```python
from build123d import *

# Parameters (mm, degrees)
SKETCH_1_R          = 28.4
EXTRUDE_1_DEPTH     = 2
SKETCH_2_R          = 13.75
EXTRUDE_2_DEPTH     = 14
SKETCH_3_R          = 3.5
SKETCH_3_R_2        = 1.6
CUT_EXTRUDE_1_DEPTH = 44.233320483
SKETCH_4_R          = 2.1
CUT_EXTRUDE_2_DEPTH = 43.533751304


with BuildPart() as part:
    # ｽｹｯﾁ1 → ﾎﾞｽ - 押し出し1 (new body)
    with BuildSketch(Plane(origin=(0, 0, 0), x_dir=(1, 0, 0), z_dir=(0, 1, 0))):
        with Locations(Location((0, 0, 0), (0, 0, 270))):
            Circle(SKETCH_1_R)
    extrude(amount=EXTRUDE_1_DEPTH)

    # ｽｹｯﾁ2 → ﾎﾞｽ - 押し出し2 (add)
    with BuildSketch(Plane(origin=(0, 2, 0), x_dir=(1, 0, 0), z_dir=(0, 1, 0))):
        with Locations(Location((0, 0, 0), (0, 0, 270))):
            Circle(SKETCH_2_R)
    extrude(amount=EXTRUDE_2_DEPTH)

    # ｽｹｯﾁ3 → ｶｯﾄ - 押し出し1 (cut, through all)
    with BuildSketch(Plane(origin=(0, 16, 0), x_dir=(1, 0, 0), z_dir=(0, 1, 0))):
        with Locations(Location((0, 0, 0), (0, 0, 270))):
            Circle(SKETCH_3_R)
        with Locations(Location((-6, 0, 0), (0, 0, 270))):
            Circle(SKETCH_3_R_2)
        with Locations(Location((6, 0, 0), (0, 0, 270))):
            Circle(SKETCH_3_R_2)
    extrude(amount=-CUT_EXTRUDE_1_DEPTH, mode=Mode.SUBTRACT)

    # ｽｹｯﾁ4 → ｶｯﾄ - 押し出し2 (cut, through all)
    with BuildSketch(Plane(origin=(0, 2, 0), x_dir=(1, 0, 0), z_dir=(0, 1, 0))):
        with Locations(Location((0, 23.4, 0), (0, 0, 270))):
            Circle(SKETCH_4_R)
        with Locations(Location((11.7, 20.264994449, 0), (0, 0, 270))):
            Circle(SKETCH_4_R)
        with Locations(Location((20.264994449, 11.7, 0), (0, 0, 270))):
            Circle(SKETCH_4_R)
        with Locations(Location((23.4, 0, 0), (0, 0, 270))):
            Circle(SKETCH_4_R)
        with Locations(Location((20.264994449, -11.7, 0), (0, 0, 270))):
            Circle(SKETCH_4_R)
        with Locations(Location((11.7, -20.264994449, 0), (0, 0, 270))):
            Circle(SKETCH_4_R)
        with Locations(Location((0, -23.4, 0), (0, 0, 270))):
            Circle(SKETCH_4_R)
        with Locations(Location((-11.7, -20.264994449, 0), (0, 0, 270))):
            Circle(SKETCH_4_R)
        with Locations(Location((-20.264994449, -11.7, 0), (0, 0, 270))):
            Circle(SKETCH_4_R)
        with Locations(Location((-23.4, 0, 0), (0, 0, 270))):
            Circle(SKETCH_4_R)
        with Locations(Location((-20.264994449, 11.7, 0), (0, 0, 270))):
            Circle(SKETCH_4_R)
        with Locations(Location((-11.7, 20.264994449, 0), (0, 0, 270))):
            Circle(SKETCH_4_R)
    extrude(amount=-CUT_EXTRUDE_2_DEPTH, mode=Mode.SUBTRACT)


solid = part.part
```
Here's how the part is built. I have some questions about the finished solid (model axes, mm). A direction names the side the tool comes from. Give positions to 0.01 mm unless a question says otherwise; leave off trailing zeros. Order: outer loops, then holes, each group sorted by start corner. A loop starts at its lowest first (then second) coordinate and runs counter-clockwise, first axis right, second up. Notation, with made-up numbers: M -13,64.5 L 24,64.5 A20 cw 24,88.5 Z; hole C -15.5,-8 d3. An arc over 180 degrees is marked long. Use a Markdown table: item, result. Add a question column.
1. Suppose I cut it at C-C (x = -12.5). List the corners of the cut face in (y, z) for me, and give its area (3 significant figures).
2. Suppose I cut it at A-A (x = 0). List the corners of the cut face in (y, z) for me, and give its area (3 significant figures).
3. For pin 1 Ø5.5 at (x, z) = (-11.7, 20.26) entering from +Y; pin 2 Ø2.5 at (x, z) = (23.4, 0) entering from -Y; pin 3 Ø2 at (x, y) = (1, 14) entering from +Z; pin 4 Ø4 at (y, z) = (5.5, 9.5) entering from -X, each with a flat end and sliding along its axis, tell me the tip position at first contact or that it passes through.
4. Suppose I cut it at B-B (z = 0). List the corners of the cut face in (x, y) for me.
5. If we mould it in two halves opening along Z, with no side actions, what happens to faces 1 (the cylindrical face through (25.17, 1.01, 1.13)), 2 (the cylindrical face through (-3.417, 8.112, -0.759)), 3 (the cylindrical face through (23.947, 0.986, 15.268)), 4 (the flat face through (0, 0, 6))? For each: +Z half, -Z half, draft (parallel to the pull), parting line (faces both ways), or undercut.
6. I need wall thicknesses on probe 1 along X at (y, z) = (0.65, 0); probe 2 along X at (y, z) = (1.55, 11.7) (3 decimals); probe 3 along X at (y, z) = (10, -0.5). Which ranges of each line are inside material? Lowest first, please. Write a range as from..to.
7. Suppose I cut it at D-D (z = -23.4). List the corners of the cut face in (x, y) for me.
8. On a 3-axis mill with a long thin cutter (end or side, diameter ignored), from which of +Z, -Z, +X, -X, +Y, -Y can I reach the whole of each face in a straight line? I mean faces 5 (the cylindrical face through (10.896, 1.014, -18.325)), 6 (the cylindrical face through (-12.2, 8.9, 6.34)). Say none if no direction works.
Results list:
| question | item | result |
|---|---|---|
| 1 | outline | M 0,-25.5 L 2,-25.5 L 2,-22.21 L 0,-22.21 Z; M 0,-18.32 L 2,-18.32 L 2,-5.73 L 16,-5.73 L 16,5.73 L 2,5.73 L 2,18.32 L 0,18.32 Z; M 0,22.21 L 2,22.21 L 2,25.5 L 0,25.5 Z |
| 1 | area | 247 mm² |
| 2 | outline | M 0,-28.4 L 2,-28.4 L 2,-25.5 L 0,-25.5 Z; M 0,-21.3 L 2,-21.3 L 2,-13.75 L 16,-13.75 L 16,-3.5 L 0,-3.5 Z; M 0,3.5 L 16,3.5 L 16,13.75 L 2,13.75 L 2,21.3 L 0,21.3 Z; M 0,25.5 L 2,25.5 L 2,28.4 L 0,28.4 Z |
| 2 | area | 370 mm² |
| 3 | pin 1 | stops at y = 2 |
| 3 | pin 2 | passes through |
| 3 | pin 3 | stops at z = 13.75 |
| 3 | pin 4 | stops at x = -11.52 |
| 4 | outline | M -28.4,0 L -25.5,0 L -25.5,2 L -28.4,2 Z; M -21.3,0 L -7.6,0 L -7.6,16 L -13.75,16 L -13.75,2 L -21.3,2 Z; M -4.4,0 L -3.5,0 L -3.5,16 L -4.4,16 Z; M 3.5,0 L 4.4,0 L 4.4,16 L 3.5,16 Z; M 7.6,0 L 21.3,0 L 21.3,2 L 13.75,2 L 13.75,16 L 7.6,16 Z; M 25.5,0 L 28.4,0 L 28.4,2 L 25.5,2 Z |
| 5 | face 1 | undercut |
| 5 | face 2 | undercut |
| 5 | face 3 | parting line |
| 5 | face 4 | draft |
| 6 | probe 1 | x = -28.4..-25.5, -21.3..-7.6, -4.4..-3.5, 3.5..4.4, 7.6..21.3, 25.5..28.4 |
| 6 | probe 2 | x = -25.878..-22.365, -18.165..18.165, 22.365..25.878 |
| 6 | probe 3 | x = -13.74..-7.52, -4.48..-3.46, 3.46..4.48, 7.52..13.74 |
| 7 | outline | M -16.09,0 L -2.1,0 L -2.1,2 L -16.09,2 Z; M 2.1,0 L 16.09,0 L 16.09,2 L 2.1,2 Z |
| 8 | face 5 | +Y, -Y |
| 8 | face 6 | +Y |
